from build123d import *

# Parameters (mm, degrees)
BOSS_EXTRU_1_DEPTH                             = 3
ESQUISSE2_W                                    = 45.5
ESQUISSE2_H                                    = 30.5
BOSS_EXTRU_2_DEPTH                             = 1.5
ESQUISSE3_W                                    = 43.5
ESQUISSE3_H                                    = 28.5
ENL_V_MAT_EXTRU_2_DEPTH                        = 2.5
FRAISAGE_POUR_VIS_T_TE_FRAIS_E_M31_D           = 3.4
FRAISAGE_POUR_VIS_T_TE_FRAIS_E_M31_CSINK_D     = 6.3
FRAISAGE_POUR_VIS_T_TE_FRAIS_E_M31_CSINK_ANGLE = 90
BOSS_EXTRU_3_START                             = 2.5
ESQUISSE6_R                                    = 2.2
ESQUISSE6_R_2                                  = 1.7
BOSS_EXTRU_3_DEPTH                             = 2.5
ENL_V_MAT_EXTRU_3_DEPTH                        = 39.194534949
FRAISAGE_POUR_VIS_T_TE_FRAIS_E_M32_D           = 3.5
FRAISAGE_POUR_VIS_T_TE_FRAIS_E_M32_CSINK_D     = 6.3
FRAISAGE_POUR_VIS_T_TE_FRAIS_E_M32_CSINK_ANGLE = 90
ENL_V_MAT_EXTRU_5_REACH                        = 40.011
ESQUISSE11_R                                   = 1.75


with BuildPart() as part:
    # Esquisse1 → Boss.-Extru.1 (new body)
    with BuildSketch(Plane.XY):
        with BuildLine():
            Line((-24.682458366, 17.5), (24.682458366, 17.5))
            ThreePointArc((24.682458366, 17.5), (30.069312487, 13.149746049), (33.65, 7.223399477))
            Line((33.65, 7.223399477), (33.65, -7.223399477))
            ThreePointArc((33.65, -7.223399477), (30.069312487, -13.149746049), (24.682458366, -17.5))
            Line((24.682458366, -17.5), (-24.682458366, -17.5))
            ThreePointArc((-24.682458366, -17.5), (-30.069312487, -13.149746049), (-33.65, -7.223399477))
            Line((-33.65, -7.223399477), (-33.65, 7.223399477))
            ThreePointArc((-33.65, 7.223399477), (-30.069312487, 13.149746049), (-24.682458366, 17.5))
        make_face()
    extrude(amount=BOSS_EXTRU_1_DEPTH)

    # Esquisse2 → Boss.-Extru.2 (add)
    with BuildSketch(Plane.XY.offset(3)):
        Rectangle(ESQUISSE2_W, ESQUISSE2_H)
    extrude(amount=BOSS_EXTRU_2_DEPTH)

    # Esquisse3 → Enlèv. mat.-Extru.2 (cut)
    with BuildSketch(Plane.XY.offset(4.5)):
        Rectangle(ESQUISSE3_W, ESQUISSE3_H)
    extrude(amount=-ENL_V_MAT_EXTRU_2_DEPTH, mode=Mode.SUBTRACT)

    # Fraisage pour vis à tête fraisée M31 (through all)
    with Locations(Plane(origin=(0, 0, 0), x_dir=(-1, 0, 0), z_dir=(0, 0, -1))):
        with Locations((-19.25, -11.75), (19.25, 11.75)):
            CounterSinkHole(FRAISAGE_POUR_VIS_T_TE_FRAIS_E_M31_D / 2, FRAISAGE_POUR_VIS_T_TE_FRAIS_E_M31_CSINK_D / 2, counter_sink_angle=FRAISAGE_POUR_VIS_T_TE_FRAIS_E_M31_CSINK_ANGLE)

    # Esquisse6 → Boss.-Extru.3 (add)
    # profile 1 of 2: a face of its own
    with BuildSketch(Plane.XY.offset(2).offset(BOSS_EXTRU_3_START)):
        with Locations((-19.25, 11.75)):
            Circle(ESQUISSE6_R)
        with Locations(Location((-19.25, 11.75, 0), (0, 0, 180))):
            Circle(ESQUISSE6_R_2, mode=Mode.SUBTRACT)
    # profile 2 of 2: a face of its own
    with BuildSketch(Plane.XY.offset(2).offset(BOSS_EXTRU_3_START)):
        with Locations((19.25, -11.75)):
            Circle(ESQUISSE6_R)
        with Locations(Location((19.25, -11.75, 0), (0, 0, 180))):
            Circle(ESQUISSE6_R_2, mode=Mode.SUBTRACT)
    extrude(amount=-BOSS_EXTRU_3_DEPTH)

    # Esquisse7 → Enlèv. mat.-Extru.3 (cut, through all)
    with BuildSketch(Plane(origin=(0, 0, 0), x_dir=(-1, 0, 0), z_dir=(0, 0, -1))):
        with BuildLine():
            Line((-27.15, 6), (-27.15, -6))
            ThreePointArc((-27.15, -6), (-28.9, -7.75), (-30.65, -6))
            Line((-30.65, -6), (-30.65, 6))
            ThreePointArc((-30.65, 6), (-28.9, 7.75), (-27.15, 6))
        make_face()
        with BuildLine():
            Line((27.15, 6), (27.15, -6))
            ThreePointArc((27.15, -6), (28.9, -7.75), (30.65, -6))
            Line((30.65, -6), (30.65, 6))
            ThreePointArc((30.65, 6), (28.9, 7.75), (27.15, 6))
        make_face()
    extrude(amount=-ENL_V_MAT_EXTRU_3_DEPTH, mode=Mode.SUBTRACT)

    # Fraisage pour vis à tête fraisée M32 (through all)
    with Locations(Plane(origin=(0, 0, 0), x_dir=(-1, 0, 0), z_dir=(0, 0, -1))):
        with Locations((-10, -10), (-10, 10)):
            CounterSinkHole(FRAISAGE_POUR_VIS_T_TE_FRAIS_E_M32_D / 2, FRAISAGE_POUR_VIS_T_TE_FRAIS_E_M32_CSINK_D / 2, counter_sink_angle=FRAISAGE_POUR_VIS_T_TE_FRAIS_E_M32_CSINK_ANGLE)

    # Esquisse11 → Enlèv. mat.-Extru.5 (cut, up to next)
    with BuildSketch(Plane.XY.offset(2), mode=Mode.PRIVATE) as enl_v_mat_extru_5_sk1:
        with Locations((-4.35, 0)):
            Circle(ESQUISSE11_R)
    enl_v_mat_extru_5_tool1 = extrude(enl_v_mat_extru_5_sk1.sketch, amount=-ENL_V_MAT_EXTRU_5_REACH, mode=Mode.PRIVATE) & part.part
    add(enl_v_mat_extru_5_tool1.solids().sort_by_distance((-4.35, 0, 2))[0], mode=Mode.SUBTRACT)


solid = part.part
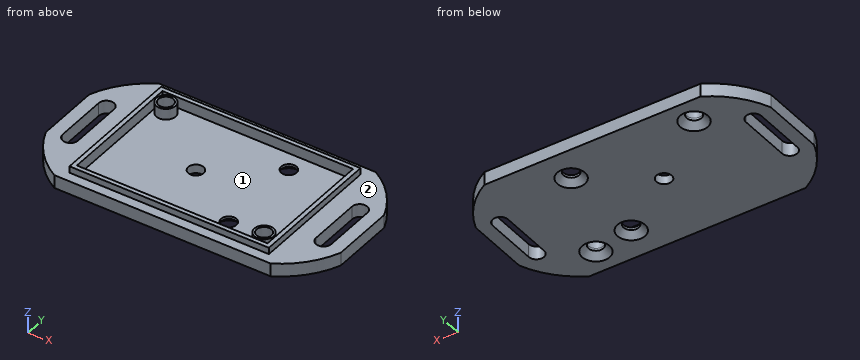
Input: part model. Units: mm. Frame: model coordinates. Face numbers are marked on the shaded views. Coordinates: 2 decimals unless noted, no trailing zeros. Loops run counter-clockwise (first coordinate to the right, second up) from the corner with the lowest first, then second, coordinate; pieces in that order, holes last.
(1) Material intervals for probe 1 along Y at (x, z) = (10, 1.6); probe 2 along Y at (x, z) = (-19.25, 3.65); probe 3 along X at (y, z) = (-2.5, 1.3), sorted ascending.
(2) Section A-A on y = 0. Return the cut outline in (x, z), then the cut area to 3 significant figures.
(3) Section D-D on x = -19.25. Return the cut outline in (y, z), then the cut area to 3 significant figures.
(4) First-contact query: pin 1 Ø8.5 at (x, y) = (-7.5, 3) entering from +Z; pin 2 Ø5.5 at (x, y) = (-19.25, 11.75) entering from -Z; pin 3 Ø1.2 at (y, z) = (-2.5, 4) entering from -X. Flat tips, straight axial feed; report the tip coordinate or a pass-through.
(5) Section B-B on x = -4.35. Return the cut outline in (y, z).
(6) Section C-C on x = 10. Return the cut outline in (y, z), then the cut area to 3 significant figures.
(7) Pull-direction query (Y, two-part tool) for the marked faces 1 and 2; classes: released by +Y, released by -Y, zero draft, split by the parting line, or undercut.
Data:
1. probe 1: y = -17.5 to -11.75, -8.25 to 8.25, 11.75 to 17.5
1. probe 2: y = -15.25 to -14.25, 9.55 to 10.05, 13.45 to 13.95, 14.25 to 15.25
1. probe 3: x = -33.65 to -30.65, -27.15 to 27.15, 30.65 to 33.65
2. outline: (-33.65, 0) - (-30.65, 0) - (-30.65, 3) - (-33.65, 3) - close; (-27.15, 0) - (-6.1, 0) - (-6.1, 2) - (-21.75, 2) - (-21.75, 4.5) - (-22.75, 4.5) - (-22.75, 3) - (-27.15, 3) - close; (-2.6, 0) - (27.15, 0) - (27.15, 3) - (22.75, 3) - (22.75, 4.5) - (21.75, 4.5) - (21.75, 2) - (-2.6, 2) - close; (30.65, 0) - (33.65, 0) - (33.65, 3) - (30.65, 3) - close
2. area: 133 mm2
3. outline: (-17.5, 0) - (8.6, 0) - (10.05, 1.45) - (10.05, 4.5) - (9.55, 4.5) - (9.55, 2) - (-14.25, 2) - (-14.25, 4.5) - (-15.25, 4.5) - (-15.25, 3) - (-17.5, 3) - close; (13.45, 1.45) - (14.9, 0) - (17.5, 0) - (17.5, 3) - (15.25, 3) - (15.25, 4.5) - (14.25, 4.5) - (14.25, 2) - (13.95, 2) - (13.95, 4.5) - (13.45, 4.5) - close
3. area: 73.1 mm2
4. pin 1: stops at z = 2
4. pin 2: stops at z = 0.4
4. pin 3: stops at x = -22.75
5. outline: (-17.5, 0) - (-1.75, 0) - (-1.75, 2) - (-14.25, 2) - (-14.25, 4.5) - (-15.25, 4.5) - (-15.25, 3) - (-17.5, 3) - close; (1.75, 0) - (17.5, 0) - (17.5, 3) - (15.25, 3) - (15.25, 4.5) - (14.25, 4.5) - (14.25, 2) - (1.75, 2) - close
6. outline: (-17.5, 0) - (-13.15, 0) - (-11.75, 1.4) - (-11.75, 2) - (-14.25, 2) - (-14.25, 4.5) - (-15.25, 4.5) - (-15.25, 3) - (-17.5, 3) - close; (-8.25, 1.4) - (-6.85, 0) - (6.85, 0) - (8.25, 1.4) - (8.25, 2) - (-8.25, 2) - close; (11.75, 1.4) - (13.15, 0) - (17.5, 0) - (17.5, 3) - (15.25, 3) - (15.25, 4.5) - (14.25, 4.5) - (14.25, 2) - (11.75, 2) - close
6. area: 61.6 mm2
7. face 1: undercut
7. face 2: zero draft
